The listing builds one solid part. Answer for the finished solid, in the listing's coordinates (mm). A direction names the side the tool comes from. Round coordinates to 2 decimals unless told otherwise and drop trailing zeros. Loops run counter-clockwise (first coordinate to the right, second up) from the corner with the lowest first, then second, coordinate; pieces in that order, holes last. Notation, with made-up numbers: M -10,-0.75 L 15,-0.75 A18 ccw 15,34.25 Z; hole C -21,86 d7. An arc over 180 degrees is marked long. Put each result on its own line as item: value. Start each with the question number.
(1) Flat-ended cylindrical pins translate along their axes: P1, Ø5, axis at x = 0.5, z = 5.5, coming from the -Y side; P2, Ø3, axis at x = -3.5, z = -6.5, coming from the +Y side. Find the tip coordinate at first contact, or state that the pin passes through.
(2) Section A-A, the plane x = 0 is taken. Determine the outline of the cut face in (y, z) (1 decimal), then the cut area to 3 significant figures.
(3) Straight lines are drawn through the part: line 1 (Y direction, x = 0, z = -5.5); line 2 (Y direction, x = 0, z = -4) (1 decimal); line 3 (Y direction, x = -3.5, z = 2) (3 decimals). For each, find the intervals that lie inside material, in ascending order.
(4) Which of the six approach directions +Z, -Z, +X, -X, +Y, -Y give full straight-line access (tool end or side, diameter ignored) to faces 5 (the face through (-3.78, 487.3, -2.9)), 6 (the face through (0, 26, 0)), 7 (the face through (0, 492.125, 0))?
(5) Determine the mould class of faces 1 (the face through (-3.51, 476.294, -4.696)), 2 (the face through (0, 0, -5)), 3 (the face through (0, 244, 9.525)), 4 (the face through (-1.032, 4.876, -4.696)) for opening direction Y: released by +Y, released by -Y, zero draft, split by the parting line, or undercut.
```python
from build123d import *

# Parameters (mm, degrees)
F1_DEPTH = 25.4
F2_R     = 4.7625
F3_DEPTH = 25.4
F5_R     = 4.7625
F6_DEPTH = 9.525


with BuildPart() as f1:
    # F0 (on Right) → F1 (new body, symmetric)
    with BuildSketch(Plane.YZ):
        Polygon((0, -9.525), (482.6, -9.525), (482.6, 0), (431.8, 0), (431.8, 9.525), (50.8, 9.525), (50.8, 0), (0, 0), align=None)
    extrude(amount=F1_DEPTH, both=True)

    # F2 (on Top) → F3 (cut)
    with BuildSketch(Plane.XY):
        with Locations((0, 9.525)):
            Circle(F2_R)
        with Locations((0, 473.075)):
            Circle(F2_R)
    extrude(amount=-F3_DEPTH, mode=Mode.SUBTRACT)

    # F5 (on offset) → F6 (join)
    with BuildSketch(Plane.XZ.offset(-482.6)):
        Circle(F5_R)
    extrude(amount=-F6_DEPTH)


solid = f1.part
```
Recorded:
1. P1: stops at y = 50.8
1. P2: stops at y = 482.6
2. outline: M 0,-9.5 L 4.8,-9.5 L 4.8,0 L 0,0 Z; M 14.3,-9.5 L 468.3,-9.5 L 468.3,0 L 431.8,0 L 431.8,9.5 L 50.8,9.5 L 50.8,0 L 14.3,0 Z; M 477.8,-9.5 L 482.6,-9.5 L 482.6,-4.8 L 492.1,-4.8 L 492.1,4.8 L 482.6,4.8 L 482.6,0 L 477.8,0 Z
2. area: 8,140 mm²
3. line 1: y = 0 to 4.76, 14.29 to 468.31, 477.84 to 482.6
3. line 2: y = 0 to 4.8, 14.3 to 468.3, 477.8 to 492.1
3. line 3: y = 50.8 to 431.8, 482.6 to 492.125
4. face 5: +Y
4. face 6: +Z, +X, -X, -Y
4. face 7: +Z, -Z, +X, -X, +Y
5. face 1: undercut
5. face 2: released by -Y
5. face 3: zero draft
5. face 4: undercut
